Can you work these out from the model? Positions are in its coordinate system, mm. Round coordinates to 2 decimals unless told otherwise and drop trailing zeros. Order: outer loops, then holes, each group sorted by start corner. A loop starts at its lowest first (then second) coordinate and runs counter-clockwise, first axis right, second up. Notation, with made-up numbers: M -16.5,49 L 42.5,49 A19 ccw 42.5,71 Z; hole C 8.25,81 d2. An arc over 180 degrees is marked long. Answer as a JSON object with one key per item and string values. Group by question number.
Autodesk Inventor part; units mm, degrees
ref_plane "YZ Plane" through (0, 0, 0) normal (1, 0, 0) x (0, 1, 0)
ref_plane "XZ Plane" through (0, 0, 0) normal (0, 1, 0) x (-1, 0, 0)
ref_plane "XY Plane" through (0, 0, 0) normal (0, 0, 1) x (1, 0, 0)
ref_plane "РабПлоскость1" through (-327.803629, 8.784154, 215.836479) normal (0, 0, 1) x (1, 0, 0)
sketch "Эскиз1" plane through (-327.803629, 8.784154, 215.836479) normal (0, 0, 1) x (1, 0, 0)
  line L0 (3.114831, 11.166777) -> (2.944416, 21.498705)
  line L1 (2.944416, 21.498705) -> (-3.054768, 21.399754)
  line L2 (-3.054768, 21.399754) -> (-2.884353, 11.067826)
  line L3 (-2.884353, 11.067826) -> (3.114831, 11.166777)
  line L4 (-3.393221, 41.919489) -> (-3.225183, 31.731682)
  line L5 (2.774001, 31.830633) -> (2.605963, 42.01844)
  line L6 (-3.225183, 31.731682) -> (2.774001, 31.830633)
  line L7 (2.605963, 42.01844) -> (-3.393221, 41.919489)
  line L8 (2.774001, 31.830633) -> (2.605963, 42.01844) construction
  line L9 (-3.393221, 41.919489) -> (-3.225183, 31.731682) construction
  line L10 (3.114831, 11.166777) -> (2.944416, 21.498705) construction
  line L11 (-3.054768, 21.399754) -> (-2.884353, 11.067826) construction
  line L12 (6.149374, 48.077701) -> (19.433282, 48.296806) construction
  line L13 (2.605963, 42.01844) -> (6.248325, 42.078517) construction
  point P0 (327.803629, -8.784154)
  dimension "d16" = 6
extrude "Выдавливание1" add sketch "Эскиз1" against normal blind 6
ref_plane "РабПлоскость2" through (-327.498735, 8.403036, 292.836479) normal (0, 0, -1) x (-0.999864, -0.0164918, 0)
sketch "Эскиз2" plane through (-327.498735, 8.403036, 292.836479) normal (0, 0, -1) x (-0.999864, -0.0164918, 0)
  line L0 (-3, 21.833317) -> (3, 21.833317)
  line L1 (3, 21.833317) -> (3, 11.499984)
  line L2 (3, 11.5) -> (-3, 11.5)
  line L3 (-3, 11.499984) -> (-3, 21.833317)
  line L4 (3, 32.16665) -> (-3, 32.16665)
  line L5 (-3, 32.16665) -> (-3, 42.355843)
  line L6 (-3, 42.5) -> (3, 42.5)
  line L7 (3, 42.355843) -> (3, 32.16665)
  line L8 (-3, 11.499984) -> (-3, 21.833317) construction
  line L9 (3, 21.833317) -> (3, 11.499984) construction
  line L10 (-3, 32.16665) -> (-3, 42.355843) construction
  line L11 (3, 42.355843) -> (3, 32.16665) construction
  point P0 (-327.315615, -13.802923)
sketch "Эскиз2 outline for Выдавливание2" plane through (-327.498735, 8.403036, 292.836479) normal (0, 0, -1) x (-0.999864, -0.0164918, 0)
  line L0 (3, 32.16665) -> (3, 42.355843)
  line L1 (-3, 32.16665) -> (3, 32.16665)
  line L2 (-3, 42.355843) -> (-3, 32.16665)
  line L3 (3, 42.355843) -> (-3, 42.355843)
  line L4 (-3, 21.833317) -> (-3, 11.499984)
  line L5 (3, 21.833317) -> (-3, 21.833317)
  line L6 (3, 11.499984) -> (3, 21.833317)
  line L7 (-3, 11.499984) -> (3, 11.499984)
extrude "Выдавливание2" add sketch "Эскиз2 outline for Выдавливание2" against normal blind 6
sketch "Эскиз3" plane through (-327.498735, 8.403036, 292.836479) normal (0, 0, -1) x (-0.999864, -0.0164918, 0)
  circle A0 centre (0, -7.644157) radius 18
  line L0 (6.642857, 42.355843) -> (3, 42.355843)
  line L1 (-3, 32.166667) -> (-3, 21.833333)
  line L2 (-3, 21.833333) -> (3, 21.833333)
  line L3 (3, 21.833333) -> (3, 32.166667)
  line L4 (3, 32.166667) -> (-3, 32.166667)
  line L5 (-3, 42.355843) -> (3, 42.355843)
  line L6 (3, 42.355843) -> (3, 10.355843)
  line L7 (3, 10.355843) -> (-3, 10.355843)
  line L8 (-3, 10.355843) -> (-3, 42.355843)
  point P0 (-327.315615, -13.802923)
  point P1 (-3, 21.833333)
  point P2 (3, 21.833333)
  point P3 (3, 42.355843)
extrude "Выдавливание3" add sketch "Эскиз3" along normal up to surface (77 mm away) contours L7 L8 L2 L6 | L2 L1 L4 L3 | L4 L8 L5 L6
sketch "Эскиз4" plane through (-331.19685, 50.703643, 209.836479) normal (-0.999864, -0.0164918, 0) x (0, 0, 1)
  line L0 (0, -14) -> (6, -14) construction
  line L1 (0, -17) -> (6, -17) construction
  line L2 (6, -17) -> (6, -14)
  line L3 (6, -14) -> (12.35, -14)
  line L4 (12.35, -14) -> (12.35, -12.75)
  line L5 (12.35, -12.75) -> (14.65, -12.75)
  line L6 (14.65, -12.75) -> (14.65, -14)
  line L7 (14.65, -14) -> (21, -14)
  line L8 (21, -14) -> (21, -17)
  line L9 (21, -17) -> (14.65, -17)
  line L10 (14.65, -17) -> (14.65, -18.25)
  line L11 (14.65, -18.25) -> (12.35, -18.25)
  line L12 (12.35, -18.25) -> (12.35, -17)
  line L13 (12.35, -17) -> (6, -17)
  line L14 (0, -20.522506) -> (0, -30.855843) construction
  line L15 (89, -10.189193) -> (89, 0) construction
  line L16 (0, -30.855843) -> (89, 0) construction
  line L17 (44.5, 0) -> (44.5, -30.855843) construction
  line L18 (89, -14) -> (83, -14) construction
  line L19 (89, -17) -> (83, -17) construction
  line L20 (83, -17) -> (83, -14)
  line L21 (83, -14) -> (76.65, -14)
  line L22 (76.65, -14) -> (76.65, -12.75)
  line L23 (76.65, -12.75) -> (74.35, -12.75)
  line L24 (74.35, -12.75) -> (74.35, -14)
  line L25 (74.35, -14) -> (68, -14)
  line L26 (68, -14) -> (68, -17)
  line L27 (68, -17) -> (74.35, -17)
  line L28 (74.35, -17) -> (74.35, -18.25)
  line L29 (74.35, -18.25) -> (76.65, -18.25)
  line L30 (76.65, -18.25) -> (76.65, -17)
  line L31 (76.65, -17) -> (83, -17)
  point P0 (-209.836479, -56.158766)
  point P1 (44.5, -15.427922)
  dimension "d9" = 2.3
  dimension "d10" = 5.5
  dimension "d11" = 15
extrude "Выдавливание4" cut sketch "Эскиз4" against normal blind 6
sketch "Эскиз5" plane through (-331.19685, 50.703643, 292.636479) normal (-0.0164918, 0.999864, 0) x (0.999864, 0.0164918, 0)
  line L0 (6, 51.133333) -> (6, 25.466667)
  line L1 (0, 51.133333) -> (6, 51.133333)
  line L2 (0, 25.466667) -> (0, 51.133333)
  line L3 (6, 25.466667) -> (0, 25.466667)
  point P0 (330.315615, 292.636479)
extrude "Выдавливание5" add sketch "Эскиз5" along normal blind 6
equation "\"d1\" = d0"
equation "\"d3\" = d0"
equation "\"d7\" = d0"
equation "\"d12\" = d3"
equation "\"d14\" = d0"
equation "\"d0\" = d16"
properties part number "Korpus 6"
1) If we section it at D-D on z = 285.5: Write out the boundary of the cut face in (x, y).
2) We'd pull the mould along Y, two halves only. Please class faces 1 (the face through (-328, 25, 209.836)), 2 (the face through (-328, 35, 277.836)): +Y half, -Y half, draft (parallel to the pull), parting line (faces both ways), or undercut.
3) If we section it at C-C on y = 25.5: Write out the boundary of the cut face in (x, z), plus the area to 3 significant figures.
4) If we section it at A-A on z = 226.5: Write out the boundary of the cut face in (x, y), plus the area to 3 significant figures.
5) I need wall thicknesses on line 1 along Y through (x, z) = (-330.25, 228); line 2 along Y through (x, z) = (-325.25, 213); line 3 along Z through (x, y) = (-326, 51.5). Which ranges of each line are inside material? Lowest first, please.
6) If we section it at B-B on z = 262: Write out the boundary of the cut face in (x, y).
7) For pin 1 (1.1 mm diameter, centred on x = -328.5, y = 31.5, fed in from -Z); pin 2 (1.5 mm diameter, centred on y = 23, z = 280.5, fed in from -X); pin 3 (1.8 mm diameter, centred on x = -326.5, y = 32, fed in from +Z), each with a flat end and sliding along its axis, tell me the tip position at first contact or that it passes through.
Findings:
{
 "1": {"outline": "M -331.2,50.7 L -330.99,37.96 L -324.99,38.05 L -325.2,50.8 Z; M -330.9,32.46 L -330.67,18.71 L -324.67,18.81 L -324.9,32.56 Z"},
 "2": {"face 1": "draft", "face 2": "undercut"},
 "3": {"outline": "M -330.78,209.84 L -324.78,209.84 L -324.78,298.84 L -330.78,298.84 Z", "area": "534 mm^2"},
 "4": {"outline": "M -331.2,50.7 L -330.97,36.71 L -324.97,36.8 L -325.2,50.8 Z; M -330.92,33.71 L -330.67,18.71 L -324.67,18.81 L -324.92,33.8 Z", "area": "174 mm^2"},
 "5": {"line 1": "y = 18.71 to 33.72, 36.72 to 50.72", "line 2": "y = 19.94 to 30.28, 40.61 to 50.8", "line 3": "z = 241.5 to 267.17"},
 "6": {"outline": "M -331.3,56.7 L -330.67,18.71 L -324.67,18.81 L -325.3,56.8 Z"},
 "7": {"pin 1": "stops at z = 215.84", "pin 2": "stops at x = -330.75", "pin 3": "stops at z = 292.84"}
}
